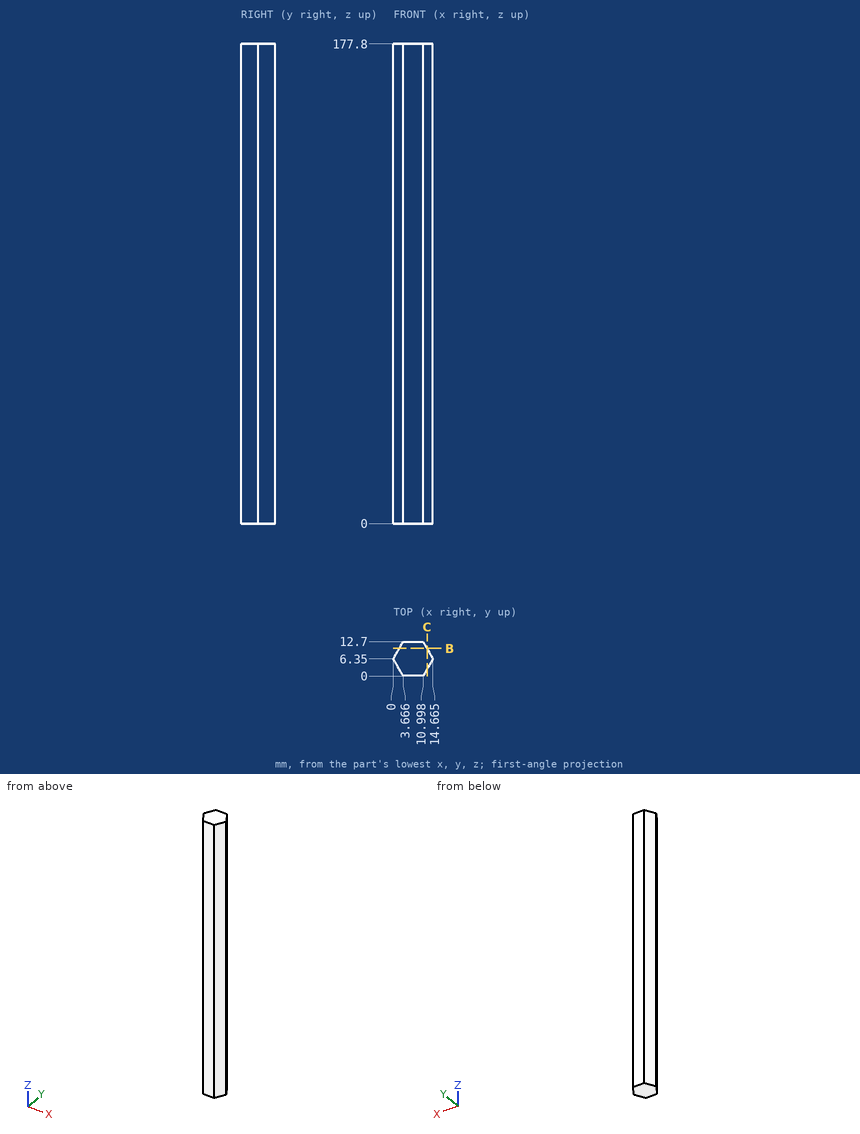
Print and shaded views of the part. All mm, measured from the part's lowest x, y and z. Give positions to 0.01 mm unless a question says otherwise; leave off trailing zeros. Order: outer loops, then holes, each group sorted by start corner. A loop starts at its lowest first (then second) coordinate and runs counter-clockwise, first axis right, second up. Notation, with made-up numbers: (-30.75, -2.75) -> (-23.75, -2.75) arc R22 ccw to (-23.75, 35.25) -> close; hole circle Ø8 at (-5.75, 22.25). An arc over 180 degrees is marked (long way). Use CSV: the item, a comma, the result in double quotes.
1. Drill centre lines: line 1 along Y through (x, z) = (13.25, 139); line 2 along Y through (x, z) = (0.5, 67) (1 decimal); line 3 along X through (y, z) = (7.25, 20.5) (1 decimal). Where is each one in solid material? Low to high. Write a range as from..to.
Outcome:
line 1,"3.9..8.8"
line 2,"5.5..7.2"
line 3,"0.5..14.1"
2. Band-saw the part on B-B, the plane y = 10.25. Give the cut face in (x, z), then the cut area to 3 significant figures.
Outcome:
outline,"(2.25, 0) -> (12.41, 0) -> (12.41, 177.8) -> (2.25, 177.8) -> close"
area,"1,810 mm²"
3. Drop a flat-ended pin along its axis: pin 1 (1.5 mm diameter, centred on y = 9, z = 30.5, fed in from -X). Give the stop position or say it passes through.
Outcome:
pin 1,"x = 1.1"
4. Band-saw the part on C-C, the plane x = 12.5. Give the cut face in (y, z), then the cut area to 3 significant figures.
Outcome:
outline,"(2.6, 0) -> (10.1, 0) -> (10.1, 177.8) -> (2.6, 177.8) -> close"
area,"1,330 mm²"
